The model under review builds one solid part; all positions refer to its coordinate system, in mm. A direction names the side the tool comes from. Coordinates: 2 decimals unless noted, no trailing zeros. Write each loop counter-clockwise with the first axis right and the second up, starting at its lowest first coordinate (ties: lowest second). Pieces come first, ordered by that corner, then holes.
```python
from build123d import *

# Parameters (mm, degrees)
F1_DEPTH = 127
F2_R     = 12.7
F3_DEPTH = 50.8
F4_DEPTH = 222.25


with BuildPart() as f1:
    # F0 (on Front) → F1 (new body)
    with BuildSketch(Plane.XZ):
        Polygon((0, 84.799479), (0, 0), (304.8, 0), (304.8, 101.6), (273.05, 101.6), (273.05, 38.1), (31.75, 38.1), (31.75, 101.6), (19.05, 101.6), align=None)
    extrude(amount=F1_DEPTH)

    # F2 (on face) → F3 (cut)
    with BuildSketch(Plane.YZ.offset(304.8)):
        with BuildLine():
            Line((-127, 101.6), (-127, 50.8))
            Line((-127, 50.8), (-107.95, 50.8))
            Line((-107.95, 50.8), (-81.305853, 94.082571))
            ThreePointArc((-81.305853, 94.082571), (-73.145897, 99.601092), (-63.5, 101.6))
            Line((-63.5, 101.6), (-127, 101.6))
        make_face()
        with BuildLine():
            Line((-19.05, 50.8), (0, 50.8))
            Line((0, 50.8), (0, 101.6))
            Line((0, 101.6), (-63.033349, 101.6))
            ThreePointArc((-63.033349, 101.6), (-53.387452, 99.601092), (-45.227496, 94.082571))
            Line((-45.227496, 94.082571), (-19.05, 50.8))
        make_face()
        Polygon((-76.2, 0), (-50.8, 0), (-50.8, 12.7), (-31.75, 12.7), (-31.75, 29.21), (-50.8, 29.21), (-50.8, 38.1), (-76.2, 38.1), (-76.2, 29.21), (-95.25, 29.21), (-95.25, 12.7), (-76.2, 12.7), align=None)
        with Locations((-63.5, 76.2)):
            Circle(F2_R)
    extrude(amount=-F3_DEPTH, mode=Mode.SUBTRACT)

    # F3_face (on face) → F4 (cut)
    with BuildSketch(Plane(origin=(254, -63.5, 19.800455), x_dir=(0, 1, 0), z_dir=(1, 0, 0))):
        Polygon((-12.7, -19.800455), (12.7, -19.800455), (12.7, -7.100455), (31.75, -7.100455), (31.75, 9.409545), (12.7, 9.409545), (12.7, 18.299545), (-12.7, 18.299545), (-12.7, 9.409545), (-31.75, 9.409545), (-31.75, -7.100455), (-12.7, -7.100455), align=None)
    extrude(amount=-F4_DEPTH, mode=Mode.SUBTRACT)


solid = f1.part
```
Item 1: Mouldability with a two-part tool opening along X and no side actions: class faces 6 (the face through (0, -63, 43)), 7 (the face through (31.75, -64, 63)), 8 (the face through (170, -31.75, 21)) as pulls with the +X half, pulls with the -X half, needs draft (parallel to the pull), parting line crosses it, or undercut.
Solved:
face 6: pulls with the -X half
face 7: undercut
face 8: needs draft
Item 2: Take a section at B-B, the plane z = 54.5. Write out the cut boundary in (x, y).
Solved:
outline: (0, -127) - (31.75, -127) - (31.75, 0) - (0, 0) - close; (273.05, -105.67) - (304.8, -105.67) - (304.8, -21.29) - (273.05, -21.29) - close
Item 3: For pin 1 (12.5 mm diameter, centred on x = 293, y = -60, fed in from -Z); pin 2 (15 mm diameter, centred on x = 289.5, y = -8, fed in from +Z); pin 3 (3 mm diameter, centred on y = -74.5, z = 26.5, fed in from +X), all flat-tipped, find the tip position at first contact; note any pin that passes through.
Solved:
pin 1: stops at z = 38.1
pin 2: stops at z = 50.8
pin 3: stops at x = 31.75
Item 4: Machinability: for faces 1 (the face through (150, -77, 0)), 2 (the face through (273.05, -63, 63)), 3 (the face through (289.147, -57.64, 64.933)), 4 (the face through (289, -10, 50.8)), 5 (the face through (289.147, -94.814, 72.138)), which of the approach directions +Z, -Z, +X, -X, +Y, -Y give a long, thin tool a straight path to every point of the face, cutting with its end or side? Answer none if there is none.
Solved:
face 1: -Z, +X, -X, +Y, -Y
face 2: +Z, +Y, -Y
face 3: +X
face 4: +Z, +X, +Y
face 5: +Z, +X, -Y
Item 5: Take a section at A-A, the plane x = 117. Write out the cut boundary in (y, z).
Solved:
outline: (-127, 0) - (-76.2, 0) - (-76.2, 12.7) - (-95.25, 12.7) - (-95.25, 29.21) - (-76.2, 29.21) - (-76.2, 38.1) - (-127, 38.1) - close; (-50.8, 0) - (0, 0) - (0, 38.1) - (-50.8, 38.1) - (-50.8, 29.21) - (-31.75, 29.21) - (-31.75, 12.7) - (-50.8, 12.7) - close
Item 6: Take a section at C-C, the plane y = -9.5. Write out the cut boundary in (x, z).
Solved:
outline: (0, 0) - (304.8, 0) - (304.8, 50.8) - (273.05, 50.8) - (273.05, 38.1) - (31.75, 38.1) - (31.75, 101.6) - (19.05, 101.6) - (0, 84.8) - close
Item 7: Take a section at D-D, the plane z = 76.2. Write out the cut boundary in (x, y), plus the area to 3 significant figures.
Solved:
outline: (0, -127) - (31.75, -127) - (31.75, 0) - (0, 0) - close; (273.05, -92.31) - (304.8, -92.31) - (304.8, -76.2) - (273.05, -76.2) - close; (273.05, -50.8) - (304.8, -50.8) - (304.8, -34.41) - (273.05, -34.41) - close
area: 5,060 mm2
Item 8: To check wall thickness, follow line 1 along X through (y, z) = (-53.5, 57); line 2 along Z through (x, y) = (290, -63.5); line 3 along Y through (x, z) = (261.5, 23). State the ranges of each line that lie inside material, in increasing order.
Solved:
line 1: x = 0 to 31.75, 273.05 to 304.8
line 2: z = 38.1 to 63.5, 88.9 to 101.6
line 3: y = -127 to -95.25, -31.75 to 0
